```python
from build123d import *

# Parameters (mm, degrees)
SKETCH2_W          = 177.8
SKETCH2_H          = 6.35
REVOLVE1_ANGLE     = 180
SKETCH3_R          = 3.327499949
CUT_EXTRUDE1_DEPTH = 175.339362144
CUT_EXTRUDE2_DEPTH = 200.191716848


with BuildPart() as part:
    # Sketch2 → Revolve1 (revolve)
    with BuildSketch(Plane(origin=(0, 0, 0), x_dir=(0, 0, -1), z_dir=(0, -1, 0))):
        with Locations((60.53129924, -60.325)):
            Rectangle(SKETCH2_W, SKETCH2_H)
    revolve(axis=Axis((0, 0, 0), (0, 0, 1)), revolution_arc=REVOLVE1_ANGLE)

    # Sketch3 → Cut-Extrude1 (cut, through all)
    with BuildSketch(Plane(origin=(0, 0, 0), x_dir=(1, 0, 0), z_dir=(0, 1, 0))):
        with Locations(Location((0, 66.88129924, 0), (0, 0, 270))):
            Circle(SKETCH3_R)
        with Locations(Location((0, 54.18129924, 0), (0, 0, 270))):
            Circle(SKETCH3_R)
        with Locations(Location((0, 79.58129924, 0), (0, 0, 270))):
            Circle(SKETCH3_R)
        with Locations(Location((0, 41.48129924, 0), (0, 0, 270))):
            Circle(SKETCH3_R)
    extrude(amount=-CUT_EXTRUDE1_DEPTH, mode=Mode.SUBTRACT)

    # Sketch4 → Cut-Extrude2 (cut, through all)
    with BuildSketch(Plane.XY.offset(28.36870076)):
        with BuildLine():
            Line((-81.567226875, -12.7), (81.567226875, -12.7))
            ThreePointArc((81.567226875, -12.7), (0, 82.55), (-81.567226875, -12.7))
        make_face()
    extrude(amount=-CUT_EXTRUDE2_DEPTH, mode=Mode.SUBTRACT)


solid = part.part
```
Input: part model. Units: mm. Frame: model coordinates. Round coordinates to 2 decimals unless told otherwise and drop trailing zeros. Loops run counter-clockwise (first coordinate to the right, second up) from the corner with the lowest first, then second, coordinate; pieces in that order, holes last. Notation, with made-up numbers: (76, 54.25) - (87, 54.25) arc R12 cw to (87, 58.25) - close; hole circle Ø1 at (9, 42.25). An arc over 180 degrees is marked (long way). One line per item, written item: value. Start each with the question number.
(1) Ray query, line 1 (Z direction, x = 0, y = -61.5); line 2 (X direction, y = -40.5, z = -24.5); line 3 (X direction, y = -52.5, z = -63.5). Return the intervals inside material, ascending. Write a range as [from, to].
(2) Section D-D, the plane x = 41. Return loops of the section in (y, z), plus the area to 3 significant figures.
(3) Section C-C, the plane z = -42. Return loops of the section in (x, y), plus the area to 3 significant figures.
(4) Draft query along Z for faces 1 (the flat face through (0, -59, 28.369)), 2 (the cylindrical face through (0.146, -60.231, -82.906)), 3 (the cylindrical face through (-1.08, -57.14, -61.78)). Return one class per face: +Z half, -Z half, draft (parallel to the pull), parting line (faces both ways), or undercut.
(5) Section A-A, the plane x = 0. Return loops of the section in (y, z).
(6) Section B-B, the plane y = -53. Return loops of the section in (x, z) (3 decimals), plus the area to 3 significant figures.
(7) Contact query for flat-ended pins moving along their axis: P1, Ø12, axis at x = 32, z = 0.5, coming from the -Y side; P2, Ø2, axis at y = -54.5, z = -76.5, coming from the +X side; P3, Ø4, axis at x = -28.5, z = 5, coming from the -Y side. Output: stop coordinate, or through.
Results below:
1. line 1: [-149.43, -82.91], [-76.25, -70.21], [-63.55, -57.51], [-50.85, -44.81], [-38.15, 28.37]
1. line 2: [-48.91, -40.32], [40.32, 48.91]
1. line 3: [-35.72, -22.58], [22.58, 35.72]
2. outline: (-48.49, -149.43) - (-39.81, -149.43) - (-39.81, 28.37) - (-48.49, 28.37) - close
2. area: 1,540 mm^2
3. outline: (-62.22, -12.7) arc R63.5 ccw to (-3.29, -63.41) - (-3.29, -57.06) arc R57.15 cw to (-55.72, -12.7) - close; (3.29, -63.41) arc R63.5 ccw to (62.22, -12.7) - (55.72, -12.7) arc R57.15 cw to (3.29, -57.06) - close
3. area: 999 mm^2
4. face 1: +Z half
4. face 2: undercut
4. face 3: draft
5. outline: (-63.5, -149.43) - (-57.15, -149.43) - (-57.15, -82.91) - (-63.5, -82.91) - close; (-63.5, -76.25) - (-57.15, -76.25) - (-57.15, -70.21) - (-63.5, -70.21) - close; (-63.5, -63.55) - (-57.15, -63.55) - (-57.15, -57.51) - (-63.5, -57.51) - close; (-63.5, -50.85) - (-57.15, -50.85) - (-57.15, -44.81) - (-63.5, -44.81) - close; (-63.5, -38.15) - (-57.15, -38.15) - (-57.15, 28.37) - (-63.5, 28.37) - close
6. outline: (-34.975, -149.431) - (-21.38, -149.431) - (-21.38, 28.369) - (-34.975, 28.369) - close; (21.38, -149.431) - (34.975, -149.431) - (34.975, 28.369) - (21.38, 28.369) - close
6. area: 4,830 mm^2
7. P1: y = -57.93
7. P2: x = 34.21
7. P3: y = -57.71
